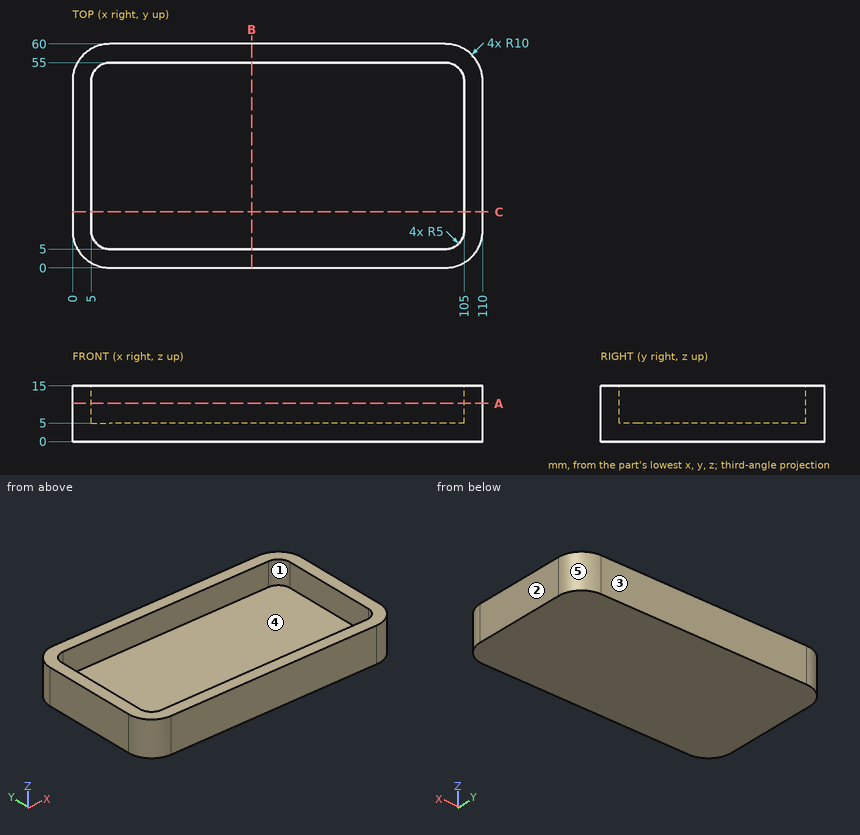
Can you work these out from the drawing? Everything is in mm from the part's minimum corner. A direction names the side the tool comes from. Round coordinates to 2 decimals unless told otherwise and drop trailing zeros. Loops run counter-clockwise (first coordinate to the right, second up) from the corner with the lowest first, then second, coordinate; pieces in that order, holes last. Notation, with made-up numbers: (16, 36) - (20, 36) arc R24 cw to (20, 54) - close; hole circle Ø2 at (-17.5, -8). An arc over 180 degrees is marked (long way). One line per question, with ' | ' between items. Start each with the question number.
Q1. I want a section at A-A (z = 10.25). Write out the boundary of the cut face in (x, y).
Q2. I want a section at B-B (x = 48). Write out the boundary of the cut face in (y, z).
Q3. I want a section at C-C (y = 15). Write out the boundary of the cut face in (x, z).
Q4. Please list where these lines run through material, in increasing order: line 1 (Y direction, x = 10, z = 9.5); line 2 (X direction, y = 30, z = 8.5); line 3 (Z direction, x = 72.5, y = 14.5). Write a range as [from, to].
Q5. We'd pull the mould along X, two halves only. Please class the marked faces 3, 4 and 5: +X half, -X half, draft (parallel to the pull), parting line (faces both ways), or undercut.
Q6. For the marked faces 1 and 2, which set-ups out of +Z, -Z, +X, -X, +Y, -Y let a thin tool reach every point of the face, with its end or its side?
Q7. Will this pin go through, and if not, where does the flat tip stop? pin 1 (3 mm diameter, centred on y = 51, z = 2.5, fed in from +X).
Response values:
1) outline: (0, 10) arc R10 ccw to (10, 0) - (100, 0) arc R10 ccw to (110, 10) - (110, 50) arc R10 ccw to (100, 60) - (10, 60) arc R10 ccw to (0, 50) - close; hole (5, 10) arc R5 ccw to (10, 5) - (100, 5) arc R5 ccw to (105, 10) - (105, 50) arc R5 ccw to (100, 55) - (10, 55) arc R5 ccw to (5, 50) - close
2) outline: (0, 0) - (60, 0) - (60, 15) - (55, 15) - (55, 5) - (5, 5) - (5, 15) - (0, 15) - close
3) outline: (0, 0) - (110, 0) - (110, 15) - (105, 15) - (105, 5) - (5, 5) - (5, 15) - (0, 15) - close
4) line 1: y = [0, 5], [55, 60] | line 2: x = [0, 5], [105, 110] | line 3: z = [0, 5]
5) face 3: draft | face 4: undercut | face 5: +X half
6) face 1: +Z | face 2: +Z, -Z, +X, +Y, -Y
7) pin 1: stops at x = 110
